```python
from build123d import *

# Parameters (mm, degrees)
SKETCH1_W           = 50
SKETCH1_H           = 30
BOSS_EXTRUDE1_DEPTH = 3
SKETCH2_W           = 3
SKETCH2_H           = 18
SKETCH2_R           = 1
BOSS_EXTRUDE2_DEPTH = 8
CHAMFER1_SIZE       = 2
FILLET1_R           = 5
CHAMFER3_SIZE       = 1


with BuildPart() as part:
    # Sketch1 → Boss-Extrude1 (new body)
    with BuildSketch(Plane.XY):
        with Locations((25, 15)):
            Rectangle(SKETCH1_W, SKETCH1_H)
    extrude(amount=BOSS_EXTRUDE1_DEPTH)

    # Sketch2 → Boss-Extrude2 (add)
    with BuildSketch(Plane.XY.offset(3)):
        with Locations((3.930461557, 9)):
            Rectangle(SKETCH2_W, SKETCH2_H)
        with Locations((19.430461557, 9)):
            Rectangle(SKETCH2_W, SKETCH2_H)
        with Locations((45, 18)):
            Circle(SKETCH2_R)
        with Locations((45, 8)):
            Circle(SKETCH2_R)
    extrude(amount=BOSS_EXTRUDE2_DEPTH)

    # Chamfer1
    chamfer1_edges = [part.edges().sort_by_distance(p)[0] for p in [
        (2.430461557, 9, 3),
        (20.930461557, 9, 3),
    ]]
    chamfer(chamfer1_edges, length=CHAMFER1_SIZE)

    # Fillet1
    fillet1_edges = [part.edges().sort_by_distance(p)[0] for p in [
        (0, 0, 1.5),
        (50, 0, 1.5),
        (50, 30, 1.5),
        (0, 30, 1.5),
    ]]
    fillet(fillet1_edges, radius=FILLET1_R)

    # Chamfer3
    chamfer3_edges = [part.edges().sort_by_distance(p)[0] for p in [
        (44, 18, 3),
        (44, 8, 3),
    ]]
    chamfer(chamfer3_edges, length=CHAMFER3_SIZE)


solid = part.part
```
Geometry check sheet. Reference: the model listing, model coordinates, mm. A direction names the side the tool comes from. Round coordinates to 2 decimals unless told otherwise and drop trailing zeros. Loops run counter-clockwise (first coordinate to the right, second up) from the corner with the lowest first, then second, coordinate; pieces in that order, holes last. Notation, with made-up numbers: (-11, 15.5) -> (1, 15.5) arc R14 cw to (1, 36.5) -> close; hole circle Ø3 at (52, 57.25). An arc over 180 degrees is marked (long way). Use a Markdown table: item, result.
(1) Sectioned sample at B-B (y = 5.5). Enter the section's corners in (x, z), then the cut area to 3 significant figures.
Calculated:
| item | result |
|---|---|
| outline | (0, 0) -> (50, 0) -> (50, 3) -> (22.93, 3) -> (20.93, 5) -> (20.93, 11) -> (17.93, 11) -> (17.93, 3) -> (5.43, 3) -> (5.43, 11) -> (2.43, 11) -> (2.43, 5) -> (0.43, 3) -> (0, 3) -> close |
| area | 202 mm² |
(2) Sectioned sample at A-A (z = 9). Enter the section's corners in (x, y).
Calculated:
| item | result |
|---|---|
| outline | (2.43, 0.71) arc R5 ccw to (5, 0) -> (5.43, 0) -> (5.43, 18) -> (2.43, 18) -> close; (17.93, 0) -> (20.93, 0) -> (20.93, 18) -> (17.93, 18) -> close; circle Ø2 at (45, 8); circle Ø2 at (45, 18) |
(3) Scan lines: probe 1 along X at (y, z) = (5.75, 5.5); probe 2 along Z at (x, y) = (26.5, 9.5); probe 3 along X at (y, z) = (15.5, 3.5). Record each from-to range of solid material in increasing order.
Calculated:
| item | result |
|---|---|
| probe 1 | 2.43 to 5.43, 17.93 to 20.93 |
| probe 2 | 0 to 3 |
| probe 3 | 0.93 to 5.43, 17.93 to 22.43 |
(4) Go/stop test with flat-tipped pins: P1, Ø6.5, axis at y = 5, z = 7.5, coming from the +X side; P2, Ø2.5, axis at y = 8, z = 7.5, coming from the -X side; P3, Ø4, axis at x = 3, z = 8.5, coming from the +Y side. Record where each tip stops, or that it passes through.
Calculated:
| item | result |
|---|---|
| P1 | x = 46 |
| P2 | x = 2.43 |
| P3 | y = 18 |
(5) Sectioned sample at D-D (y = 25.5). Enter the section's corners in (x, z), then the cut area to 3 significant figures.
Calculated:
| item | result |
|---|---|
| outline | (0.03, 0) -> (49.97, 0) -> (49.97, 3) -> (0.03, 3) -> close |
| area | 150 mm² |
(6) Sectioned sample at C-C (x = 38.5). Enter the section's corners in (y, z), then the cut area to 3 significant figures.
Calculated:
| item | result |
|---|---|
| outline | (0, 0) -> (30, 0) -> (30, 3) -> (0, 3) -> close |
| area | 90.0 mm² |
(7) Mould release check, pull along Y, two halves, no side actions. Record for faces 1 (the cylindrical face through (46, 8, 7)), 2 (the flat face through (1.44, 9.23, 4.01)), 3 (the flat face through (4, 18, 7)): released by +Y, released by -Y, zero draft, split by the parting line, or undercut.
Calculated:
| item | result |
|---|---|
| face 1 | undercut |
| face 2 | zero draft |
| face 3 | released by +Y |
(8) Set-up check for faces 4 (the flat face through (45, 8, 11)), 5 (the flat face through (21.92, 8.87, 4.01)), 6 (the flat face through (2.43, 9, 8)): record each of +Z, -Z, +X, -X, +Y, -Y from which the full face is reachable in a straight line by a thin tool's end or side.
Calculated:
| item | result |
|---|---|
| face 4 | +Z, +X, -X, +Y, -Y |
| face 5 | +Z, +Y, -Y |
| face 6 | +Z, -X, +Y, -Y |
